Model file for the job. Use its own axes, mm. Coordinates: 2 decimals unless noted, no trailing zeros. Write each loop counter-clockwise with the first axis right and the second up, starting at its lowest first coordinate (ties: lowest second). Pieces come first, ordered by that corner, then holes. Notation, with made-up numbers: M 4,31.5 L 14,31.5 A13 ccw 14,42.5 Z; hole C 6,2.5 d10. An arc over 180 degrees is marked long. Answer in a Markdown table with one row per item. Add a question column.
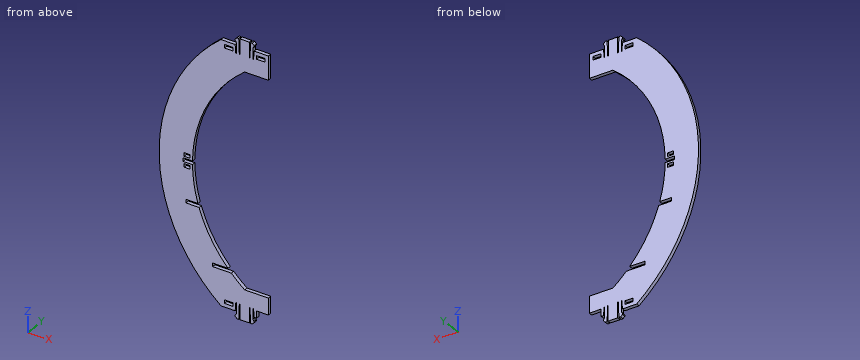
```python
from build123d import *

# Parameters (mm, degrees)
BOSS_EXTRUDE2_DEPTH      = 3
SKETCH3_W                = 10
SKETCH3_H                = 6
SKETCH3_W_2              = 7
SKETCH3_H_2              = 3
CUT_EXTRUDE1_DEPTH       = 3
CUT_EXTRUDE3_DEPTH       = 1
CUT_EXTRUDE3_DEPTH_BACK  = 3
SKETCH10_W               = 5
SKETCH10_H               = 3
CUT_EXTRUDE4_DEPTH       = 10
CUT_EXTRUDE12_DEPTH      = 1
CUT_EXTRUDE12_DEPTH_BACK = 3
CUT_EXTRUDE13_DEPTH      = 1
CUT_EXTRUDE13_DEPTH_BACK = 3


with BuildPart() as part:
    # Sketch2 → Boss-Extrude2 (new body)
    with BuildSketch(Plane(origin=(0, 0, 0), x_dir=(1, 0, 0), z_dir=(0, 1, 0))):
        with BuildLine():
            Line((-70, 90), (-50, 90))
            Line((-50, 90), (-50, 110))
            Line((-50, 110), (-61.99554496, 110))
            Line((-61.99554496, 110), (-62.49554496, 102.997828908))
            Line((-62.49554496, 102.997828908), (-62.99554496, 102.997828908))
            Line((-62.99554496, 102.997828908), (-62.99554496, 111.997828908))
            Line((-62.99554496, 111.997828908), (-62.49554496, 112.997828908))
            Line((-62.49554496, 112.997828908), (-61.99554496, 113.497828908))
            Line((-61.99554496, 113.497828908), (-61.99554496, 114.497828908))
            Line((-61.99554496, 114.497828908), (-63.49554496, 115.997828908))
            Line((-63.49554496, 115.997828908), (-64.99554496, 115.997828908))
            Line((-64.99554496, 115.997828908), (-65.49554496, 102.997828908))
            Line((-65.49554496, 102.997828908), (-65.99554496, 102.997828908))
            Line((-65.99554496, 102.997828908), (-65.99554496, 115.997828908))
            Line((-65.99554496, 115.997828908), (-73.99554496, 115.997828908))
            Line((-73.99554496, 115.997828908), (-73.99554496, 102.997828908))
            Line((-73.99554496, 102.997828908), (-74.49554496, 102.997828908))
            Line((-74.49554496, 102.997828908), (-74.99554496, 115.997828908))
            Line((-74.99554496, 115.997828908), (-76.49554496, 115.997828908))
            Line((-76.49554496, 115.997828908), (-77.99554496, 114.497828908))
            Line((-77.99554496, 114.497828908), (-77.99554496, 113.497828908))
            Line((-77.99554496, 113.497828908), (-77.49554496, 112.997828908))
            Line((-77.49554496, 112.997828908), (-76.99554496, 111.997828908))
            Line((-76.99554496, 111.997828908), (-76.99554496, 102.997828908))
            Line((-76.99554496, 102.997828908), (-77.49554496, 102.997828908))
            Line((-77.49554496, 102.997828908), (-77.99554496, 110))
            Line((-77.99554496, 110), (-90, 110))
            ThreePointArc((-90, 110), (-142.126704036, 0), (-90, -110))
            Line((-90, -110), (-78.00445504, -110))
            Line((-78.00445504, -110), (-77.50445504, -102.997828908))
            Line((-77.50445504, -102.997828908), (-77.00445504, -102.997828908))
            Line((-77.00445504, -102.997828908), (-77.00445504, -111.997828908))
            Line((-77.00445504, -111.997828908), (-77.50445504, -112.997828908))
            Line((-77.50445504, -112.997828908), (-78.00445504, -113.497828908))
            Line((-78.00445504, -113.497828908), (-78.00445504, -114.497828908))
            Line((-78.00445504, -114.497828908), (-76.50445504, -115.997828908))
            Line((-76.50445504, -115.997828908), (-75.00445504, -115.997828908))
            Line((-75.00445504, -115.997828908), (-74.50445504, -102.997828908))
            Line((-74.50445504, -102.997828908), (-74.00445504, -102.997828908))
            Line((-74.00445504, -102.997828908), (-74.00445504, -115.997828908))
            Line((-74.00445504, -115.997828908), (-66.00445504, -115.997828908))
            Line((-66.00445504, -115.997828908), (-66.00445504, -102.997828908))
            Line((-66.00445504, -102.997828908), (-65.50445504, -102.997828908))
            Line((-65.50445504, -102.997828908), (-65.00445504, -115.997828908))
            Line((-65.00445504, -115.997828908), (-63.50445504, -115.997828908))
            Line((-63.50445504, -115.997828908), (-62.00445504, -114.497828908))
            Line((-62.00445504, -114.497828908), (-62.00445504, -113.497828908))
            Line((-62.00445504, -113.497828908), (-62.50445504, -112.997828908))
            Line((-62.50445504, -112.997828908), (-63.00445504, -111.997828908))
            Line((-63.00445504, -111.997828908), (-63.00445504, -102.997828908))
            Line((-63.00445504, -102.997828908), (-62.50445504, -102.997828908))
            Line((-62.50445504, -102.997828908), (-62.00445504, -110))
            Line((-62.00445504, -110), (-50, -110))
            Line((-50, -110), (-50, -90))
            Line((-50, -90), (-70, -90))
            ThreePointArc((-70, -90), (-114.01754251, 0), (-70, 90))
        make_face()
    extrude(amount=BOSS_EXTRUDE2_DEPTH)

    # Sketch3 → Cut-Extrude1 (cut)
    with BuildSketch(Plane(origin=(0, 3, 0), x_dir=(1, 0, 0), z_dir=(0, 1, 0))):
        with Locations((-55, 107)):
            Rectangle(SKETCH3_W, SKETCH3_H)
        with Locations((-83.5, 105.5)):
            Rectangle(SKETCH3_W_2, SKETCH3_H_2)
        with Locations((-56.491089921, -105.5)):
            Rectangle(SKETCH3_W_2, SKETCH3_H_2)
        with Locations((-83.491089921, -105.5)):
            Rectangle(SKETCH3_W_2, SKETCH3_H_2)
    extrude(amount=-CUT_EXTRUDE1_DEPTH, mode=Mode.SUBTRACT)

    # Sketch8 → Cut-Extrude3 (cut, two sides)
    with BuildSketch(Plane(origin=(0, 3, 0), x_dir=(1, 0, 0), z_dir=(0, 1, 0))) as cut_extrude3_sk:
        Polygon((163.594434528, 1.5), (-114.00767518, 1.5), (-122.00767518, 1.5), (-122.00767518, -1.5), (-114.00767518, -1.5), (163.594434528, -1.5), (718.798653945, -1.5), (718.798653945, 1.5), align=None)
    extrude(amount=CUT_EXTRUDE3_DEPTH, mode=Mode.SUBTRACT)
    extrude(cut_extrude3_sk.sketch, amount=-CUT_EXTRUDE3_DEPTH_BACK, mode=Mode.SUBTRACT)

    # Sketch10 → Cut-Extrude4 (cut)
    with BuildSketch(Plane(origin=(0, 3, 0), x_dir=(1, 0, 0), z_dir=(0, 1, 0))):
        with Locations((-118.50767518, 4.5)):
            Rectangle(SKETCH10_W, SKETCH10_H)
        with Locations((-118.50767518, -4.5)):
            Rectangle(SKETCH10_W, SKETCH10_H)
    extrude(amount=-CUT_EXTRUDE4_DEPTH, mode=Mode.SUBTRACT)

    # Sketch9 → Cut-Extrude12 (cut, two sides)
    with BuildSketch(Plane(origin=(0, 3, 0), x_dir=(1, 0, 0), z_dir=(0, 1, 0))) as cut_extrude12_sk:
        Polygon((339.233941087, 80), (-81.240384046, 80), (-97.089238313, 80), (-97.089238313, 77), (-84.089238313, 77), (336.385086821, 77), (946.188662062, -502.080505639), (949.037516328, -499.080505639), align=None)
    extrude(amount=CUT_EXTRUDE12_DEPTH, mode=Mode.SUBTRACT)
    extrude(cut_extrude12_sk.sketch, amount=-CUT_EXTRUDE12_DEPTH_BACK, mode=Mode.SUBTRACT)

    # Sketch13 → Cut-Extrude13 (cut, two sides)
    with BuildSketch(Plane(origin=(0, 3, 0), x_dir=(1, 0, 0), z_dir=(0, 1, 0))) as cut_extrude13_sk:
        Polygon((225.364323888, 35), (-108.512672071, 35), (-119.434912162, 35), (-119.434912162, 32), (-109.434912162, 32), (224.442083797, 32), (862.717356055, -164.214348471), (863.639596146, -161.214348471), align=None)
    extrude(amount=CUT_EXTRUDE13_DEPTH, mode=Mode.SUBTRACT)
    extrude(cut_extrude13_sk.sketch, amount=-CUT_EXTRUDE13_DEPTH_BACK, mode=Mode.SUBTRACT)


solid = part.part
```
1) Flat gauge pins, fed straight in: pin 1 Ø0.9 at (y, z) = (1.5, -105.5) entering from +X; pin 2 Ø0.9 at (x, y) = (-85.5, 2) entering from +Z; pin 3 Ø1.5 at (y, z) = (2, -79) entering from +X; pin 4 Ø5 at (x, z) = (-93, -84) entering from -Y. Where does each tip first touch, or does it go through?
2) Slice it at A-A (y = 1.75). Count the separate pieces of the cut face and the enclosed holes in it, then the cut area to 3 significant figures.
3) Drill centre lines: probe 1 along Z at (x, y) = (-54.5, 2.75); probe 2 along Z at (x, y) = (-96.5, 1.2); probe 3 along Z at (x, y) = (-81, 0.8). Where is each one in solid material? Low to high.
4) Slice it at B-B (z = 8.5). Give the cut face in (x, y).
5) Slice it at C-C (x = -128). Give the cut face in (y, z).
Ans:
| question | item | result |
|---|---|---|
| 1 | pin 1 | stops at x = -60 |
| 1 | pin 2 | stops at z = 110 |
| 1 | pin 3 | stops at x = -97.09 |
| 1 | pin 4 | stops at y = 0 |
| 2 | separate pieces | 1 |
| 2 | enclosed holes | 5 |
| 2 | area | 7,520 mm2 |
| 3 | probe 1 | z = -104 to -90, 90 to 104, 107 to 110 |
| 3 | probe 2 | z = -104.34 to -80, -77 to -60.73, 60.73 to 104.34 |
| 3 | probe 3 | z = -110 to -107, -104 to -80.24, 80.24 to 104, 107 to 110 |
| 4 | outline | M -141.87,0 L -113.7,0 L -113.7,3 L -141.87,3 Z |
| 5 | outline | M 0,-61.77 L 3,-61.77 L 3,61.77 L 0,61.77 Z |
